Can you work these out from the model? Positions are in its coordinate system, mm. A direction names the side the tool comes from. Coordinates: 2 decimals unless noted, no trailing zeros. Loops run counter-clockwise (first coordinate to the right, second up) from the corner with the lowest first, then second, coordinate; pieces in that order, holes last. Notation, with made-up numbers: (21.25, -1.5) -> (38.25, -1.5) arc R19 cw to (38.25, 33.5) -> close; hole circle Ø9 at (42, 47). An arc over 180 degrees is marked (long way). Put each result on its own line as item: value. Start each with the question number.
Item 1: Will these pins go through, and if not, where does the flat tip stop? P1, Ø3.5, axis at x = -1.5, z = 15, coming from the -Y side; P2, Ø0.8, axis at x = 19.5, y = 30.5, coming from the +Z side.
Item 2: If we section it at A-A on z = -0.5: Please give me the cut outline in (x, y).
Item 3: Please list where these lines run through material, in increasing order: L1, parallel to Z at x = -14, y = 16; L2, parallel to Z at x = 9.5, y = 151. Write a range as from..to.
Item 4: If we section it at C-C on x = 0.5: State how many separate pieces and enclosed holes the cut face has, plus the area to 3 significant figures.
Item 5: We'd pull the mould along X, two halves only. Please class faces 4 (the flat face through (0, 90, 19)), 5 (the flat face through (0, 181, 18.5)): pulls with the +X half, pulls with the -X half, needs draft (parallel to the pull), parting line crosses it, or undercut.
Item 6: If we section it at B-B on y = 85: Please give me the cut outline in (x, z).
Item 7: For faces 1 (the flat face through (0, 101, 20)), 2 (the flat face through (0, 50, 19)), 3 (the flat face through (0, 141, 18.5)), which set-ups out of +Z, -Z, +X, -X, +Y, -Y let a thin tool reach every point of the face, with its end or its side?
Autodesk Inventor part; units mm, degrees
ref_plane "YZ Plane" through (0, 0, 0) normal (1, 0, 0) x (0, 1, 0)
ref_plane "XZ Plane" through (0, 0, 0) normal (0, 1, 0) x (-1, 0, 0)
ref_plane "XY Plane" through (0, 0, 0) normal (0, 0, 1) x (1, 0, 0)
sketch "Sketch1" plane through (0, 0, 0) normal (0, 1, 0) x (-1, 0, 0)
  line L0 (20, 20) -> (-20, 20)
  line L1 (-20, 20) -> (-20, -20)
  line L2 (-20, -20) -> (20, -20)
  line L3 (20, -20) -> (20, 20)
  line L4 (20, 20) -> (-20, -20) construction
  line L5 (-20, 20) -> (20, -20) construction
  line L6 (-18.5, 18.5) -> (18.5, 18.5)
  line L7 (18.5, 18.5) -> (18.5, -18.5)
  line L8 (18.5, -18.5) -> (-18.5, -18.5)
  line L9 (-18.5, -18.5) -> (-18.5, 18.5)
  point P0 (0, 0)
  dimension "d7" = 40
  dimension "d8" = 40
  dimension "d9" = 1.5
extrude "Extrusion1" add sketch "Sketch1" along normal blind 200
sketch "Sketch2" plane through (20, 0, 20) normal (1, 0, 0) x (0, 0, -1)
  line L0 (0, 0) -> (0, 200)
  line L1 (0, 30) -> (7, 30)
  line L2 (7, 30) -> (7, 31.5)
  line L3 (7, 31.5) -> (0, 31.5)
  line L4 (0, 31.5) -> (0, 30)
  point P0 (20, 0)
  point P1 (0, 31.5)
  dimension "d10" = 7
  dimension "d11" = 1.5
  dimension "d17" = 30
extrude "Extrusion2" cut sketch "Sketch2" against normal through all
pattern_linear "Rectangular Pattern1" count 49 spacing 20 along (0, 1, 0) of "Extrusion2"
sketch "Sketch5" plane through (0, 0, 0) normal (1, 0, 0) x (0, 1, 0)
  line L0 (0, 20) -> (0, -20)
  line L1 (0, 20) -> (30, 20)
  line L2 (0, -20) -> (0.007, 20)
  line L3 (200, -20) -> (200, 20)
  line L4 (0, -20) -> (200, -20)
  line L5 (200, 20) -> (199.993, -20)
  point P0 (0, 0)
  dimension "d18" = 0.01
extrude "Extrusion3" [suppressed]
equation "\"d1\" = BEAM_5_lenth"
equation "\"d18\" = BEAM_5_angle"
properties part number "MNT-CDF-315 beam 5"
Solutions:
1. P1: through
1. P2: z = 13
2. outline: (-20, 0) -> (-18.5, 0) -> (-18.5, 200) -> (-20, 200) -> close; (18.5, 0) -> (20, 0) -> (20, 200) -> (18.5, 200) -> close
3. L1: -20..-18.5, 18.5..20
3. L2: -20..-18.5
4. separate pieces: 11
4. enclosed holes: 0
4. area: 580 mm^2
5. face 4: needs draft
5. face 5: undercut
6. outline: (-20, -20) -> (20, -20) -> (20, 20) -> (-20, 20) -> close; hole (-18.5, -18.5) -> (18.5, -18.5) -> (18.5, 18.5) -> (-18.5, 18.5) -> close
7. face 1: +Z, +X, -X, +Y, -Y
7. face 2: +Z, +X, -X
7. face 3: +Y, -Y
